```python
from build123d import *

# Parameters (mm, degrees)
SKETCH1_R           = 127
BOSS_EXTRUDE1_DEPTH = 12.7
SKETCH2_R           = 12.7
CUT_EXTRUDE2_DEPTH  = 12.7
SKETCH4_R           = 88.9
BOSS_EXTRUDE2_DEPTH = 39.6875
CHAMFER2_SIZE2      = 57.124100733
CHAMFER2_SIZE       = 39.6875
SKETCH6_R           = 31.775899267
BOSS_EXTRUDE3_DEPTH = 36.5125
SKETCH7_R           = 19.05
CUT_EXTRUDE3_DEPTH  = 155.3845


with BuildPart() as part:
    # Sketch1 → Boss-Extrude1 (new body)
    with BuildSketch(Plane(origin=(0, 0, 0), x_dir=(1, 0, 0), z_dir=(0, 1, 0))):
        with Locations(Location((0, 0, 0), (0, 0, 270))):
            Circle(SKETCH1_R)
    extrude(amount=BOSS_EXTRUDE1_DEPTH)

    # Sketch2 → Cut-Extrude2 (cut)
    with BuildSketch(Plane(origin=(0, 12.7, 0), x_dir=(1, 0, 0), z_dir=(0, 1, 0))):
        with Locations(Location((0, 107.95, 0), (0, 0, 270))):
            Circle(SKETCH2_R)
        with Locations(Location((0, -107.95, 0), (0, 0, 270))):
            Circle(SKETCH2_R)
        with Locations(Location((-93.6625, 53.975, 0), (0, 0, 270))):
            Circle(SKETCH2_R)
        with Locations(Location((93.6625, 53.975, 0), (0, 0, 270))):
            Circle(SKETCH2_R)
        with Locations(Location((-93.6625, -53.975, 0), (0, 0, 270))):
            Circle(SKETCH2_R)
        with Locations(Location((93.6625, -53.975, 0), (0, 0, 270))):
            Circle(SKETCH2_R)
    extrude(amount=-CUT_EXTRUDE2_DEPTH, mode=Mode.SUBTRACT)

    # Sketch4 → Boss-Extrude2 (add)
    with BuildSketch(Plane(origin=(0, 12.7, 0), x_dir=(1, 0, 0), z_dir=(0, 1, 0))):
        with Locations(Location((0, 0, 0), (0, 0, 90))):
            Circle(SKETCH4_R)
    extrude(amount=BOSS_EXTRUDE2_DEPTH)

    # Chamfer2
    chamfer2_edges = [part.edges().sort_by_distance(p)[0] for p in [
        (0, 52.3875, 88.9),
    ]]
    chamfer2_side = [part.faces().sort_by_distance(p)[0] for p in [
        (0, 51.59375, 88.9),
    ]]
    chamfer(chamfer2_edges, length=CHAMFER2_SIZE - 0.0001, length2=CHAMFER2_SIZE2 - 0.0001, reference=chamfer2_side[0])  # a hair under: the kernel refuses the full size

    # Sketch6 → Boss-Extrude3 (add)
    with BuildSketch(Plane(origin=(0, 52.3875, 0), x_dir=(1, 0, 0), z_dir=(0, 1, 0))):
        with Locations(Location((0, 0, 0), (0, 0, 270))):
            Circle(SKETCH6_R)
    extrude(amount=BOSS_EXTRUDE3_DEPTH)

    # Sketch7 → Cut-Extrude3 (cut)
    with BuildSketch(Plane(origin=(0, 88.9, 0), x_dir=(1, 0, 0), z_dir=(0, 1, 0))):
        with Locations(Location((0, 0, 0), (0, 0, 270))):
            Circle(SKETCH7_R)
    extrude(amount=-CUT_EXTRUDE3_DEPTH, mode=Mode.SUBTRACT)


solid = part.part
```
Work out the finished part from the listing and answer in its coordinate system (mm). A direction names the side the tool comes from. Give positions to 0.01 mm unless a question says otherwise; leave off trailing zeros. Write each loop counter-clockwise with the first axis right and the second up, starting at its lowest first coordinate (ties: lowest second). Pieces come first, ordered by that corner, then holes. Notation, with made-up numbers: (-34, 62.25) - (-6, 62.25) arc R22 ccw to (-6, 85.25) - close; hole circle Ø7 at (-13.5, -10). An arc over 180 degrees is marked (long way). Use one line per item in the form item = value.
1. Determine the mould class of faces 3 (the face through (-26, 0, -2)), 4 (the face through (-11.59, 45.07, -15.12)), 5 (the face through (-28.19, 70.39, 14.66)) for opening direction X: released by +X, released by -X, zero draft, split by the parting line, or undercut.
Filled in:
face_3 = zero draft
face_4 = undercut
face_5 = split by the parting line
2. A cutting plane is placed at C-C (y = 58). Write down the section's boundary in (x, z), and give its area (3 significant figures).
Filled in:
outline = circle Ø63.55 at (0, 0); hole circle Ø38.1 at (0, 0)
area = 2,030 mm^2
3. A cutting plane is placed at A-A (x = 0). State how many separate pieces and enclosed holes the cut face has, and give its area (3 significant figures).
Filled in:
separate_pieces = 4
enclosed_holes = 0
area = 6,300 mm^2
4. Consider L1, parallel to X at y = 11.5, z = 53.5; L2, parallel to Z at x = -1, y = 6; L3, parallel to Y at x = -18, z = -98. Determine where each line is inside the solid, lowest interval first.
Filled in:
L1 = -115.18 to -106.35, -80.97 to 80.97, 106.35 to 115.18
L2 = -127 to -120.61, -95.29 to -19.02, 19.02 to 95.29, 120.61 to 127
L3 = 0 to 12.7
5. For faces 1 (the face through (85, 12.7, -38)), 2 (the face through (102.246, 6.439, -63.335)), determine the directions among +Z, -Z, +X, -X, +Y, -Y from which every point of the face is accessible in a straight line to the end or side of a thin tool.
Filled in:
face_1 = +Y
face_2 = +Y, -Y
6. Each of these flat-tipped pins is pushed along its axis until it touches: pin 1 Ø3 at (x, z) = (87, 96) entering from +Y; pin 2 Ø8 at (x, y) = (-0.5, 33) entering from +Z; pin 3 Ø10 at (y, z) = (32.5, 33) entering from +X; pin 4 Ø5 at (x, z) = (39.5, 29.5) entering from +Y. Where does it stop, or does it pass through?
Filled in:
pin_1 = through
pin_2 = 65.44
pin_3 = 59.44
pin_4 = 41.95
7. A cutting plane is placed at D-D (z = -107.95). Write down the section's boundary in (x, y), and give its area (3 significant figures).
Filled in:
outline = (-66.9, 0) - (-12.7, 0) - (-12.7, 12.7) - (-66.9, 12.7) - close; (12.7, 0) - (66.9, 0) - (66.9, 12.7) - (12.7, 12.7) - close
area = 1,380 mm^2
